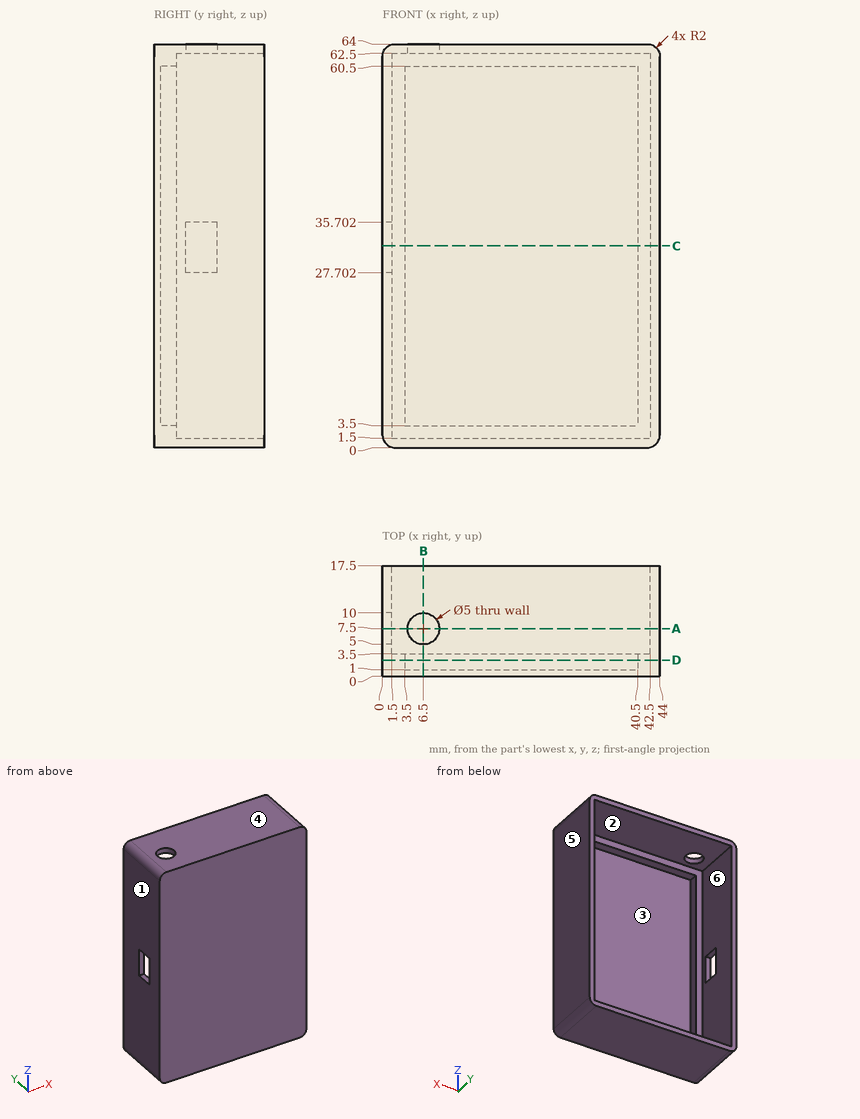
Design review of the part shown in the three views and the two pictorial views. Dimensions are in mm from the part's minimum x, y and z. A direction names the side the tool comes from. Give positions to 0.01 mm unless a question says otherwise; leave off trailing zeros. Write each loop counter-clockwise with the first axis right and the second up, starting at its lowest first coordinate (ties: lowest second). Pieces come first, ordered by that corner, then holes. Notation, with made-up numbers: M 58,88.5 L 94,88.5 A11 cw 94,92.5 Z; hole C 25,-20.75 d8. An arc over 180 degrees is marked long. Return JSON: item names as keys, results as strings. Group by question number.
Item 1: Tool access review of the marked faces 5 and 6: name each direction out of +Z, -Z, +X, -X, +Y, -Y from which nothing blocks a thin tool from reaching the whole face with its end or side.
Item 2: The part is to be moulded in two halves that separate along Z. For the marked faces 1, 2, 3 and 4, say which applies: pulls with the +Z half, pulls with the -Z half, needs draft (parallel to the pull), parting line crosses it, or undercut.
Item 3: Wall thickness on line 1 along Z through (x, y) = (23.5, 8.75); line 2 along X through (y, z) = (8, 5); line 3 along Y through (x, z) = (6.5, 63.5): over which ranges is each line inside the solid? List them lowest first.
Item 4: Clearance check with flat-ended pins moving along their axes: pin 1 Ø0.8 at (x, y) = (1, 7.5) entering from -Z; pin 2 Ø11 at (x, z) = (27, 39) entering from +Y; pin 3 Ø10 at (x, z) = (7, 54) entering from +Y. State where each tip first meets the part, or that it passes through.
Item 5: Take a section at B-B (x = 6.5). Give the boundary of the cut face in (y, z).
Item 6: Take a section at A-A (y = 7.5). Give the boundary of the cut face in (x, z).
Item 7: Take a section at C-C (z = 32). Give the boundary of the cut face in (x, y), plus the area to 3 significant figures.
Item 8: Take a section at D-D (y = 2.5). Give the boundary of the cut face in (x, z).
Return value:
{
 "1": {"face 5": "+Z, -Z, +X, +Y, -Y", "face 6": "+Y"},
 "2": {"face 1": "needs draft", "face 2": "undercut", "face 3": "undercut", "face 4": "pulls with the +Z half"},
 "3": {"line 1": "z = 0 to 1.5, 62.5 to 64", "line 2": "x = 0 to 1.5, 42.5 to 44", "line 3": "y = 0 to 5, 10 to 17.5"},
 "4": {"pin 1": "stops at z = 0.09", "pin 2": "stops at y = 1", "pin 3": "stops at y = 3.5"},
 "5": {"outline": "M 0,0 L 17.5,0 L 17.5,1.5 L 3.5,1.5 L 3.5,3.5 L 1,3.5 L 1,60.5 L 3.5,60.5 L 3.5,62.5 L 5,62.5 L 5,64 L 0,64 Z; M 10,62.5 L 17.5,62.5 L 17.5,64 L 10,64 Z"},
 "6": {"outline": "M 0,2 A2 ccw 2,0 L 42,0 A2 ccw 44,2 L 44,62 A2 ccw 42,64 L 9,64 L 9,62.5 L 42.5,62.5 L 42.5,1.5 L 1.5,1.5 L 1.5,27.7 L 0,27.7 Z; M 0,35.7 L 1.5,35.7 L 1.5,62.5 L 4,62.5 L 4,64 L 2,64 A2 ccw 0,62 Z"},
 "7": {"outline": "M 0,0 L 44,0 L 44,17.5 L 42.5,17.5 L 42.5,3.5 L 40.5,3.5 L 40.5,1 L 3.5,1 L 3.5,3.5 L 1.5,3.5 L 1.5,5 L 0,5 Z; M 0,10 L 1.5,10 L 1.5,17.5 L 0,17.5 Z", "area": "96.0 mm2"},
 "8": {"outline": "M 0,2 A2 ccw 2,0 L 42,0 A2 ccw 44,2 L 44,62 A2 ccw 42,64 L 2,64 A2 ccw 0,62 Z; hole M 3.5,3.5 L 40.5,3.5 L 40.5,60.5 L 3.5,60.5 Z"}
}
